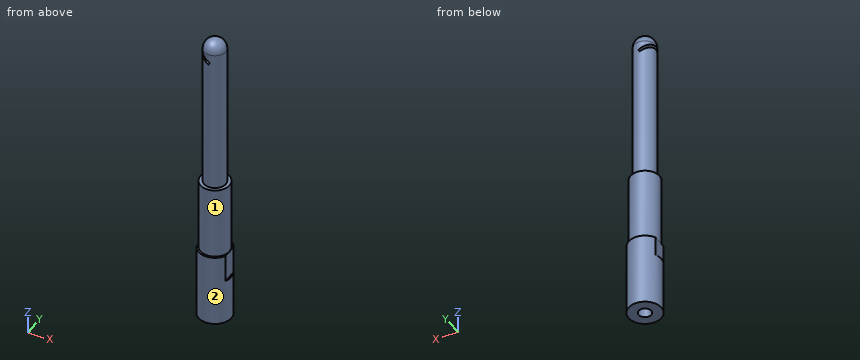
```python
from build123d import *

# Parameters (mm, degrees)
F2_W          = 3
F2_H          = 11
F3_DEPTH      = 9.001
F3_DEPTH_BACK = 9.001
F4_W          = 3
F4_H          = 16
F5_DEPTH      = 9.001
F5_DEPTH_BACK = 9.001
F7_DEPTH      = 9.001
F7_DEPTH_BACK = 9.001


with BuildPart() as f1:
    # F0 (on Front) → F1 (revolve)
    with BuildSketch(Plane.XZ):
        with BuildLine():
            Line((-9, 0), (-3.5, 0))
            Line((-3.5, 0), (-3.5, 160))
            Line((-3.5, 160), (0, 162))
            Line((0, 162), (0, 166))
            ThreePointArc((0, 166), (-4.2426406871, 164.2426406871), (-6, 160))
            Line((-6, 160), (-6, 80))
            Line((-6, 80), (-8, 80))
            Line((-8, 80), (-8, 40))
            Line((-8, 40), (-9, 40))
            Line((-9, 40), (-9, 0))
        make_face()
    revolve(axis=Axis((0, 0, 83), (0, 0, -1)))

    # F2 (on Front) → F3 (cut, two sides)
    with BuildSketch(Plane.XZ) as f3_sk:
        with Locations((-9.5278133973, 34.973811388)):
            Rectangle(F2_W, F2_H)
    extrude(amount=-F3_DEPTH, mode=Mode.SUBTRACT)
    extrude(f3_sk.sketch, amount=F3_DEPTH_BACK, mode=Mode.SUBTRACT)

    # F4 (on Front) → F5 (cut, two sides)
    with BuildSketch(Plane.XZ) as f5_sk:
        with Locations((9.5230324529, 32.8434021473)):
            Rectangle(F4_W, F4_H)
    extrude(amount=-F5_DEPTH, mode=Mode.SUBTRACT)
    extrude(f5_sk.sketch, amount=F5_DEPTH_BACK, mode=Mode.SUBTRACT)

    # F6 (on Front) → F7 (cut, two sides)
    with BuildSketch(Plane.XZ) as f7_sk:
        Polygon((-8.3235528891, 160.1148097822), (-9.0406632825, 158.7973301111), (-0.2574654756, 154.0165941548), (0.4596449178, 155.3340738258), align=None)
    extrude(amount=F7_DEPTH, mode=Mode.SUBTRACT)
    extrude(f7_sk.sketch, amount=-F7_DEPTH_BACK, mode=Mode.SUBTRACT)


solid = f1.part
```
The model under review builds one solid part; all positions refer to its coordinate system, in mm. Face numbers are marked on the shaded views. A direction names the side the tool comes from. Round coordinates to 2 decimals unless told otherwise and drop trailing zeros. Order: outer loops, then holes, each group sorted by start corner. A loop starts at its lowest first (then second) coordinate and runs counter-clockwise, first axis right, second up.
(1) For P1, Ø9, axis at y = 0.5, z = 36, coming from the +X side; P2, Ø1.5, axis at y = 5.5, z = 18.5, coming from the -X side; P3, Ø2, axis at x = -1, y = -0.5, coming from the +Z side, all flat-tipped, find the tip position at first contact; note any pin that passes through.
Working result:
P1: stops at x = 8.02
P2: stops at x = -7.64
P3: stops at z = 166
(2) Take a section at A-A, the plane z = 31.5. State the section outline as (x, y) points, plus the area to 3 significant figures.
Working result:
outline: (-8.03, -4.07) arc R9 ccw to (8.02, -4.08) - (8.02, 4.08) arc R9 ccw to (-8.03, 4.07) - close; hole circle Ø7 at (0, 0)
area: 205 mm2
(3) Wall thickness on L1, parallel to Y at x = 0, z = 69.5; L2, parallel to Y at x = 0, z = 118.5; L3, parallel to X at y = 0.25, z = 12: over which ranges is each line inside the solid? List them lowest first.
Working result:
L1: y = -8 to -3.5, 3.5 to 8
L2: y = -6 to -3.5, 3.5 to 6
L3: x = -9 to -3.49, 3.49 to 9
(4) Tool access review of the marked faces 1 and 2: name each direction out of +Z, -Z, +X, -X, +Y, -Y from which nothing blocks a thin tool from reaching the whole face with its end or side.
Working result:
face 1: +Z
face 2: +Z, -Z
(5) Take a section at C-C, the plane z = 81.5. State the section outline as (x, y) points.
Working result:
outline: circle Ø12 at (0, 0); hole circle Ø7 at (0, 0)
(6) Take a section at B-B, the plane z = 53. State the section outline as (x, y) points, plus the area to 3 significant figures.
Working result:
outline: circle Ø16 at (0, 0); hole circle Ø7 at (0, 0)
area: 163 mm2
